Part model, mm, in its own coordinate system. Give positions to 0.01 mm unless a question says otherwise; leave off trailing zeros. Order: outer loops, then holes, each group sorted by start corner. A loop starts at its lowest first (then second) coordinate and runs counter-clockwise, first axis right, second up. Notation, with made-up numbers: M 87,46.5 L 118,46.5 A13 cw 118,68.5 Z; hole C -19,-32 d9. An arc over 180 degrees is marked long. Return JSON: item names as keys, results as strings.
from build123d import *

# Parameters (mm, degrees)
SKETCH1_W           = 165.1
SKETCH1_H           = 165.1
BOSS_EXTRUDE1_DEPTH = 3.75
CUT_EXTRUDE1_REACH  = 118.804
SKETCH2_R           = 4.25
CUT_EXTRUDE2_REACH  = 118.804


with BuildPart() as part:
    # Sketch1 → Boss-Extrude1 (new body)
    with BuildSketch(Plane(origin=(0, 0, 0), x_dir=(1, 0, 0), z_dir=(0, 1, 0))):
        Rectangle(SKETCH1_W, SKETCH1_H)
    extrude(amount=BOSS_EXTRUDE1_DEPTH)

    # Sketch2 → Cut-Extrude1 (cut, up to next)
    with BuildSketch(Plane(origin=(0, 3.75, 0), x_dir=(1, 0, 0), z_dir=(0, 1, 0)), mode=Mode.PRIVATE) as cut_extrude1_sk1:
        with Locations(Location((69.85, 63.5, 0), (0, 0, 270))):
            Circle(SKETCH2_R)
    cut_extrude1_tool1 = extrude(cut_extrude1_sk1.sketch, amount=-CUT_EXTRUDE1_REACH, mode=Mode.PRIVATE) & part.part
    # Sketch2 → Cut-Extrude1 (cut, up to next)
    with BuildSketch(Plane(origin=(0, 3.75, 0), x_dir=(1, 0, 0), z_dir=(0, 1, 0)), mode=Mode.PRIVATE) as cut_extrude1_sk2:
        with Locations(Location((-57.15, 63.5, 0), (0, 0, 270))):
            Circle(SKETCH2_R)
    cut_extrude1_tool2 = extrude(cut_extrude1_sk2.sketch, amount=-CUT_EXTRUDE1_REACH, mode=Mode.PRIVATE) & part.part
    # Sketch2 → Cut-Extrude1 (cut, up to next)
    with BuildSketch(Plane(origin=(0, 3.75, 0), x_dir=(1, 0, 0), z_dir=(0, 1, 0)), mode=Mode.PRIVATE) as cut_extrude1_sk3:
        with Locations(Location((-57.15, -63.5, 0), (0, 0, 270))):
            Circle(SKETCH2_R)
    cut_extrude1_tool3 = extrude(cut_extrude1_sk3.sketch, amount=-CUT_EXTRUDE1_REACH, mode=Mode.PRIVATE) & part.part
    # Sketch2 → Cut-Extrude1 (cut, up to next)
    with BuildSketch(Plane(origin=(0, 3.75, 0), x_dir=(1, 0, 0), z_dir=(0, 1, 0)), mode=Mode.PRIVATE) as cut_extrude1_sk4:
        with Locations(Location((69.85, -63.5, 0), (0, 0, 270))):
            Circle(SKETCH2_R)
    cut_extrude1_tool4 = extrude(cut_extrude1_sk4.sketch, amount=-CUT_EXTRUDE1_REACH, mode=Mode.PRIVATE) & part.part
    add(cut_extrude1_tool1.solids().sort_by_distance((69.85, 3.75, -63.5))[0], mode=Mode.SUBTRACT)
    add(cut_extrude1_tool2.solids().sort_by_distance((-57.15, 3.75, -63.5))[0], mode=Mode.SUBTRACT)
    add(cut_extrude1_tool3.solids().sort_by_distance((-57.15, 3.75, 63.5))[0], mode=Mode.SUBTRACT)
    add(cut_extrude1_tool4.solids().sort_by_distance((69.85, 3.75, 63.5))[0], mode=Mode.SUBTRACT)

    # Sketch3 → Cut-Extrude2 (cut, up to next)
    with BuildSketch(Plane.XZ, mode=Mode.PRIVATE) as cut_extrude2_sk1:
        with BuildLine():
            Line((-67.55, -20), (-67.55, 20))
            ThreePointArc((-67.55, 20), (-61.692135624, 34.142135624), (-47.55, 40))
            Line((-47.55, 40), (47.55, 40))
            ThreePointArc((47.55, 40), (61.692135624, 34.142135624), (67.55, 20))
            Line((67.55, 20), (67.55, -20))
            ThreePointArc((67.55, -20), (61.692135624, -34.142135624), (47.55, -40))
            Line((47.55, -40), (-47.55, -40))
            ThreePointArc((-47.55, -40), (-61.692135624, -34.142135624), (-67.55, -20))
        make_face()
    cut_extrude2_tool1 = extrude(cut_extrude2_sk1.sketch, amount=-CUT_EXTRUDE2_REACH, mode=Mode.PRIVATE) & part.part
    add(cut_extrude2_tool1.solids().sort_by_distance((0, 0, 0))[0], mode=Mode.SUBTRACT)


solid = part.part
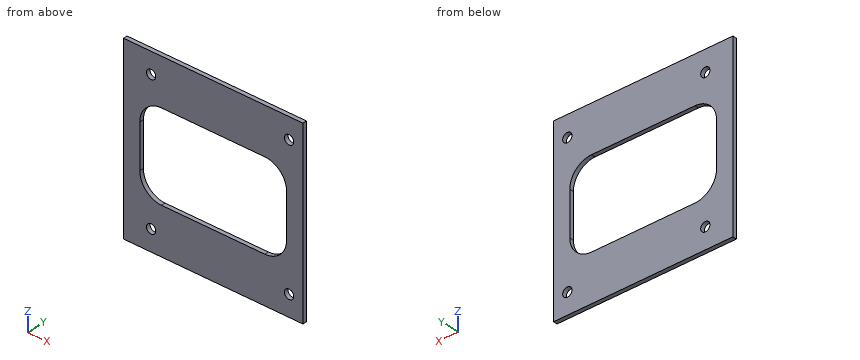
Q1. Band-saw the part on D-D (z = 4.5). Give the cut face in (x, y).
Established:
{"outline": "M -82.55,0 L -67.55,0 L -67.55,3.75 L -82.55,3.75 Z; M 67.55,0 L 82.55,0 L 82.55,3.75 L 67.55,3.75 Z"}
Q2. Band-saw the part on B-B (x = -43.5). Give the cut face in (y, z), then the cut area to 3 significant figures.
Established:
{"outline": "M 0,-82.55 L 3.75,-82.55 L 3.75,-40 L 0,-40 Z; M 0,40 L 3.75,40 L 3.75,82.55 L 0,82.55 Z", "area": "319 mm²"}
Q3. Band-saw the part on C-C (x = 69.85). Give the cut face in (y, z).
Established:
{"outline": "M 0,-82.55 L 3.75,-82.55 L 3.75,-67.75 L 0,-67.75 Z; M 0,-59.25 L 3.75,-59.25 L 3.75,59.25 L 0,59.25 Z; M 0,67.75 L 3.75,67.75 L 3.75,82.55 L 0,82.55 Z"}
Q4. Probe line 1 along X through (y, z) = (2.25, -63.5); line 2 along X through (y, z) = (1.3, -10.5); line 3 along Z through (x, y) = (-15, 0.2). List the from-to ranges inside material, lowest first.
Established:
{"line 1": "x = -82.55 to -61.4, -52.9 to 65.6, 74.1 to 82.55", "line 2": "x = -82.55 to -67.55, 67.55 to 82.55", "line 3": "z = -82.55 to -40, 40 to 82.55"}
Q5. Band-saw the part on A-A (z = 63.5). Give the cut face in (x, y).
Established:
{"outline": "M -82.55,0 L -61.4,0 L -61.4,3.75 L -82.55,3.75 Z; M -52.9,0 L 65.6,0 L 65.6,3.75 L -52.9,3.75 Z; M 74.1,0 L 82.55,0 L 82.55,3.75 L 74.1,3.75 Z"}
